Part model, mm, in its own coordinate system. Coordinates: 2 decimals unless noted, no trailing zeros.
```python
from build123d import *

# Parameters (mm, degrees)
PAD013_DEPTH                = 3
CYLINDER043_R               = 1.75
CYLINDER043_DEPTH           = 18
CYLINDER043_ROLL_ANGLE      = -89.999776
CYLINDER043_PITCH_ANGLE     = 1.4e-05
CYLINDER043_PLACEMENT_ANGLE = -9.999925
CYLINDER041_R               = 3
CYLINDER041_DEPTH           = 3
CYLINDER041_ROLL_ANGLE      = -89.999776
CYLINDER041_PITCH_ANGLE     = 1.4e-05
CYLINDER041_PLACEMENT_ANGLE = -9.999925


with BuildPart() as obj1:
    # Sketch013 → Pad013 (new body)
    with BuildSketch(Plane.XY):
        with BuildLine():
            add(Edge.make_bspline(
                [(44.997663, -28.408983), (45.245046, -6.764399), (28.5, -0.316434)],
                knots=[1.556693, 1.556693, 1.556693, 2.83913, 2.83913, 2.83913], degree=2, weights=[1, 0.801368, 1]))
            Line((28.5, -0.316434), (28.5, -25.5))
            Line((28.5, -25.5), (44.997663, -28.408983))
        make_face()
    extrude(amount=PAD013_DEPTH)


with BuildPart() as obj1_1:
    # Body015 placement: moved
    add(obj1.part.moved(Location((0, 0, 28))))


with BuildPart() as cylinder043:
    # Cylinder043 → Cylinder043 (new body)
    with BuildSketch(Plane.XY):
        Circle(CYLINDER043_R)
    extrude(amount=CYLINDER043_DEPTH)


with BuildPart() as cylinder043_1:
    # Cylinder043 roll: moved
    add(cylinder043.part.rotate(Axis((0, 0, 0), (1, 0, 0)), CYLINDER043_ROLL_ANGLE))


with BuildPart() as cylinder043_2:
    # Cylinder043 pitch: moved
    add(cylinder043_1.part.rotate(Axis((0, 0, 0), (0, 1, 0)), CYLINDER043_PITCH_ANGLE))


with BuildPart() as cylinder043_3:
    # Cylinder043 placement: moved
    add(cylinder043_2.part.moved(Location((32.058057, -23.765835, 25.500009))).rotate(Axis((32.058057, -23.765835, 25.500009), (0, 0, 1)), CYLINDER043_PLACEMENT_ANGLE))


with BuildPart() as cut059:
    # Cylinder041 → Cylinder041 (new body)
    with BuildSketch(Plane.XY):
        Circle(CYLINDER041_R)
    extrude(amount=CYLINDER041_DEPTH)


with BuildPart() as cut059_1:
    # Cylinder041 roll: moved
    add(cut059.part.rotate(Axis((0, 0, 0), (1, 0, 0)), CYLINDER041_ROLL_ANGLE))


with BuildPart() as cut059_2:
    # Cylinder041 pitch: moved
    add(cut059_1.part.rotate(Axis((0, 0, 0), (0, 1, 0)), CYLINDER041_PITCH_ANGLE))


with BuildPart() as cut059_3:
    # Cylinder041 placement: moved
    add(cut059_2.part.moved(Location((34.14182, -11.94814, 25.500056))).rotate(Axis((34.14182, -11.94814, 25.500056), (0, 0, 1)), CYLINDER041_PLACEMENT_ANGLE))

    # Cut039: cut Cylinder043
    add(cylinder043_3.part, mode=Mode.SUBTRACT)

    # Cut059: cut obj1
    add(obj1_1.part, mode=Mode.SUBTRACT)


solid = cut059_3.part
```
(1) Drop flat-ended pins along their axis: pin 1 (2 mm diameter, centred on x = 36.5, y = -11.5, fed in from -Z); pin 2 (2 mm diameter, centred on y = -10.5, z = 24, fed in from -X). Give the stop position or say it passes through.
(2) Probe line 1 (Z direction, x = 32.75, y = -10.7); line 2 (X direction, y = -10.85, z = 25.4); line 3 (Z direction, x = 34.75, y = -11.4). List the from-to ranges inside material, lowest first.
(3) Pull direction Z, two halves, no side cores. Call faces 1 (the face through (35.194, -10.632, 27.053)), 2 (the face through (34.5, -10.5, 22.5)), 3 (the face through (34, -10, 28)): +Z half, -Z half, draft (parallel to the pull), parting line (faces both ways), or undercut.
Here are the results:
1. pin 1: stops at z = 22.77
1. pin 2: stops at x = 31.33
2. line 1: z = 22.95 to 24.76, 26.24 to 28
2. line 2: x = 31.29 to 32.56, 36.11 to 37.38
2. line 3: z = 22.54 to 23.82, 27.18 to 28
3. face 1: undercut
3. face 2: parting line
3. face 3: +Z half
